Read the model definition and answer for the solid it produces. Units are mm, in the model's axes. Coordinates: 2 decimals unless noted, no trailing zeros. Loops run counter-clockwise (first coordinate to the right, second up) from the corner with the lowest first, then second, coordinate; pieces in that order, holes last. Notation, with made-up numbers: (18, 89) -> (62, 89) arc R12 cw to (62, 98) -> close; hole circle Ø7 at (69.5, -13). An arc over 180 degrees is marked (long way). Answer as a JSON object with one key per item and string values. Group by question number.
1) Section C-C, the plane x = -54.5 is taken. Give the vertices of the cut face in (y, z).
2) Section B-B, the plane x = 66.5 is taken. Give the vertices of the cut face in (y, z), plus the area to 3 significant figures.
3) Section A-A, the plane y = 20 is taken. Give the vertices of the cut face in (x, z).
4) Consider probe 1 along Y at (x, z) = (66.5, 1); probe 2 along X at (y, z) = (-20.5, 0.1); probe 3 along X at (y, z) = (-20, 1.3). Determine where each line is inside the solid, lowest interval first. Write a range as [from, to].
from build123d import *

# Parameters (mm, degrees)
SKETCH_W                = 139
SKETCH_H                = 46
PAD_DEPTH               = 2
SKETCH001_R             = 2
POCKET_DEPTH            = 294.855913
SKETCH001_MIRRORED_2_R  = 2
POCKET_MIRRORED_2_DEPTH = 294.855913
POCKET001_DEPTH         = 2.001


with BuildPart() as part:
    # Sketch → Pad (new body)
    with BuildSketch(Plane.XY):
        Rectangle(SKETCH_W, SKETCH_H)
    extrude(amount=PAD_DEPTH)

    # Sketch001 (on Face6 of Pad) → Pocket (cut, through all)
    with BuildSketch(Plane.XY.offset(2)):
        with Locations((-66.5, 20)):
            Circle(SKETCH001_R)
    pocket = extrude(amount=-POCKET_DEPTH, mode=Mode.SUBTRACT)

    # Sketch001 Mirrored 2 → Pocket Mirrored 2 (cut, through all)
    with BuildSketch(Plane(origin=(0, 0, 2), x_dir=(-1, 0, 0), z_dir=(0, 0, -1))):
        with Locations((-66.5, 20)):
            Circle(SKETCH001_MIRRORED_2_R)
    pocket_mirrored_2 = extrude(amount=POCKET_MIRRORED_2_DEPTH, mode=Mode.SUBTRACT)

    # Mirrored001: Pocket, Pocket Mirrored 2 across Sketch001 H_Axis
    add(pocket.mirror(Plane(origin=(0, 0, 2), x_dir=(0, 0, 1), z_dir=(0, 1, 0))), mode=Mode.SUBTRACT)
    add(pocket_mirrored_2.mirror(Plane(origin=(0, 0, 2), x_dir=(0, 0, 1), z_dir=(0, 1, 0))), mode=Mode.SUBTRACT)

    # Sketch002 (on Face5 of MultiTransform) → Pocket001 (cut, through all)
    with BuildSketch(Plane.XY.offset(2)):
        with BuildLine():
            ThreePointArc((-50.5, -23), (-54.5, -19), (-58.5, -23))
            Line((-58.5, -23), (-50.5, -23))
        make_face()
    extrude(amount=-POCKET001_DEPTH, mode=Mode.SUBTRACT)


solid = part.part
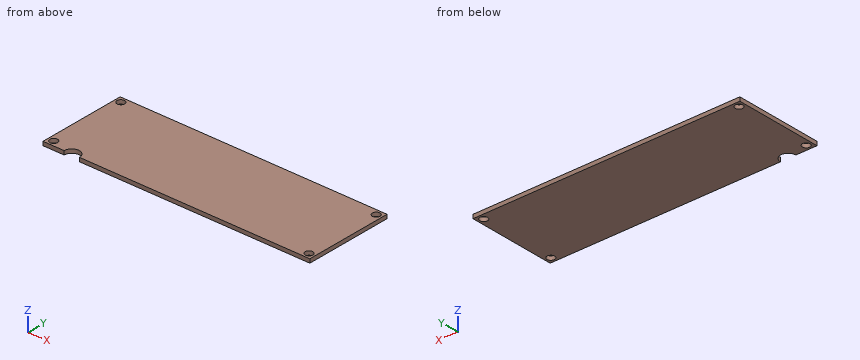
Determined:
{
 "1": {"outline": "(-19, 0) -> (23, 0) -> (23, 2) -> (-19, 2) -> close"},
 "2": {"outline": "(-23, 0) -> (-22, 0) -> (-22, 2) -> (-23, 2) -> close; (-18, 0) -> (18, 0) -> (18, 2) -> (-18, 2) -> close; (22, 0) -> (23, 0) -> (23, 2) -> (22, 2) -> close", "area": "76.0 mm²"},
 "3": {"outline": "(-69.5, 0) -> (-68.5, 0) -> (-68.5, 2) -> (-69.5, 2) -> close; (-64.5, 0) -> (64.5, 0) -> (64.5, 2) -> (-64.5, 2) -> close; (68.5, 0) -> (69.5, 0) -> (69.5, 2) -> (68.5, 2) -> close"},
 "4": {"probe 1": "[-23, -22], [-18, 18], [22, 23]", "probe 2": "[-69.5, -68.44], [-64.56, -57.62], [-51.38, 64.56], [68.44, 69.5]", "probe 3": "[-69.5, -68.5], [-64.5, -57.15], [-51.85, 64.5], [68.5, 69.5]"}
}
